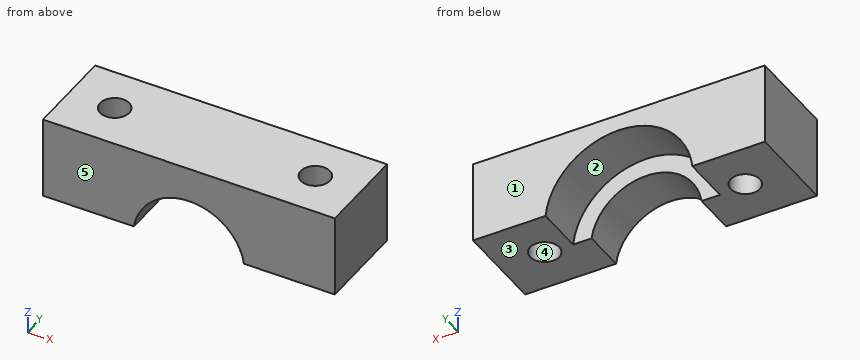
from build123d import *

# Parameters (mm, degrees)
SKETCH1_W           = 32
SKETCH1_H           = 27
SKETCH1_R           = 1.5
BOSS_EXTRUDE1_DEPTH = 25
SKETCH3_W           = 20
SKETCH3_H           = 10
SKETCH3_H_2         = 7
CUT_EXTRUDE1_DEPTH  = 33
SKETCH4_R           = 6.1
CUT_EXTRUDE6_DEPTH  = 18
SKETCH5_R           = 8.1
CUT_EXTRUDE7_DEPTH  = 5.3
SKETCH7_R           = 1.6
CUT_EXTRUDE8_DEPTH  = 26
CUT_EXTRUDE9_DEPTH  = 10
SKETCH10_W          = 32
SKETCH10_H          = 27
CUT_EXTRUDE10_DEPTH = 16


with BuildPart() as part:
    # Sketch1 → Boss-Extrude1 (new body)
    with BuildSketch(Plane.XY):
        with Locations((16, -13.5)):
            Rectangle(SKETCH1_W, SKETCH1_H)
        with Locations((8.5, -3.5)):
            Circle(SKETCH1_R, mode=Mode.SUBTRACT)
        with Locations((23.5, -3.5)):
            Circle(SKETCH1_R, mode=Mode.SUBTRACT)
        with Locations((8.5, -23.5)):
            Circle(SKETCH1_R, mode=Mode.SUBTRACT)
        with Locations((23.5, -23.5)):
            Circle(SKETCH1_R, mode=Mode.SUBTRACT)
    extrude(amount=BOSS_EXTRUDE1_DEPTH)

    # Sketch3 → Cut-Extrude1 (cut, through all)
    with BuildSketch(Plane.ZY):
        with Locations((15, -5)):
            Rectangle(SKETCH3_W, SKETCH3_H)
        with Locations((15, -23.5)):
            Rectangle(SKETCH3_W, SKETCH3_H_2)
    extrude(amount=-CUT_EXTRUDE1_DEPTH, mode=Mode.SUBTRACT)

    # Sketch4 → Cut-Extrude6 (cut, through all)
    with BuildSketch(Plane(origin=(0, -10, 0), x_dir=(1, 0, 0), z_dir=(0, 1, 0))):
        with Locations((15.999687497, -15.1)):
            Circle(SKETCH4_R)
    extrude(amount=-CUT_EXTRUDE6_DEPTH, mode=Mode.SUBTRACT)

    # Sketch5 → Cut-Extrude7 (cut)
    with BuildSketch(Plane(origin=(0, -10, 0), x_dir=(1, 0, 0), z_dir=(0, 1, 0))):
        with Locations((15.999687497, -15.1)):
            Circle(SKETCH5_R)
    extrude(amount=-CUT_EXTRUDE7_DEPTH, mode=Mode.SUBTRACT)

    # Sketch7 → Cut-Extrude8 (cut, through all)
    with BuildSketch(Plane.XY.offset(25)):
        with Locations((5, -15)):
            Circle(SKETCH7_R)
        with Locations((27, -15)):
            Circle(SKETCH7_R)
    extrude(amount=-CUT_EXTRUDE8_DEPTH, mode=Mode.SUBTRACT)

    # Sketch9 → Cut-Extrude9 (cut)
    with BuildSketch(Plane(origin=(0, 0, 0), x_dir=(-1, 0, 0), z_dir=(0, 0, -1))):
        Polygon((-29.138778877, -12.825574808), (-29.952496893, -15.765024245), (-27.813718016, -17.939449437), (-24.861221123, -17.174425192), (-24.047503107, -14.234975755), (-26.186281984, -12.060550563), align=None)
        Polygon((-5, -11.95), (-7.641377482, -13.475), (-7.641377482, -16.525), (-5, -18.05), (-2.358622518, -16.525), (-2.358622518, -13.475), align=None)
    extrude(amount=-CUT_EXTRUDE9_DEPTH, mode=Mode.SUBTRACT)

    # Sketch10 → Cut-Extrude10 (cut)
    with BuildSketch(Plane(origin=(0, 0, 0), x_dir=(-1, 0, 0), z_dir=(0, 0, -1))):
        with Locations((-16, -13.5)):
            Rectangle(SKETCH10_W, SKETCH10_H)
    extrude(amount=-CUT_EXTRUDE10_DEPTH, mode=Mode.SUBTRACT)


solid = part.part
The listing builds one solid part. Answer for the finished solid, in the listing's coordinates (mm). Face numbers are marked on the shaded views. A direction names the side the tool comes from. Round coordinates to 2 decimals unless told otherwise and drop trailing zeros. Write each loop counter-clockwise with the first axis right and the second up, starting at its lowest first coordinate (ties: lowest second). Pieces come first, ordered by that corner, then holes. Notation, with made-up numbers: M 6,40 L 37,40 A20 cw 37,68 Z; hole C -29,0 d8. An arc over 180 degrees is marked long. Write each question's results on one line, items separated by ' | '. Start each with the question number.
Item 1: For a pull along Y with two mould halves and no side action, classify the marked faces 3, 4 and 5 as pulls with the +Y half, pulls with the -Y half, needs draft (parallel to the pull), parting line crosses it, or undercut.
Item 2: For the marked faces 1 and 2, determine the directions among +Z, -Z, +X, -X, +Y, -Y from which every point of the face is accessible in a straight line to the end or side of a thin tool.
Item 3: A flat-ended cylindrical pin translates along its axis: pin 1 Ø3.5 at (x, z) = (17, 19) entering from +Y. Find the tip coordinate at first contact, or state that the pin passes through.
Item 4: A cutting plane is placed at A-A on x = 5. Write down the section's boundary in (y, z), and give its area (3 significant figures).
Item 5: A cutting plane is placed at C-C on y = -13. Write down the section's boundary in (x, z), and give its area (3 significant figures).
Item 6: A cutting plane is placed at B-B on z = 20.5. Write down the section's boundary in (x, y).
Item 7: Straight lines are drawn through the part: L1, parallel to Y at x = 27, z = 21.25; L2, parallel to X at y = -15.75, z = 18; L3, parallel to X at y = -11.5, z = 20.5. For each, find the intervals that lie inside material, in ascending order. Write a range as [from, to].
Item 8: A cutting plane is placed at D-D on z = 22. Write down the section's boundary in (x, y), and give its area (3 significant figures).
Check sheet entries:
1) face 3: needs draft | face 4: undercut | face 5: pulls with the -Y half
2) face 1: +Z, -Z, +X, -X, +Y | face 2: -Z, +Y
3) pin 1: through
4) outline: M -20,16 L -16.6,16 L -16.6,25 L -20,25 Z; M -13.4,16 L -10,16 L -10,25 L -13.4,25 Z | area: 61.2 mm²
5) outline: M 0,16 L 7.95,16 A8.1 cw 24.05,16 L 32,16 L 32,25 L 0,25 Z | area: 199 mm²
6) outline: M 0,-20 L 13.16,-20 L 13.16,-15.3 L 9.96,-15.3 L 9.96,-10 L 0,-10 Z; M 18.84,-20 L 32,-20 L 32,-10 L 22.04,-10 L 22.04,-15.3 L 18.84,-15.3 Z; hole C 5,-15 d3.2; hole C 27,-15 d3.2
7) L1: [-20, -16.6], [-13.4, -10] | L2: [0, 3.59], [6.41, 10.63], [21.37, 25.59], [28.41, 32] | L3: [0, 9.96], [22.04, 32]
8) outline: M 0,-20 L 32,-20 L 32,-10 L 20.24,-10 L 20.24,-15.3 L 11.76,-15.3 L 11.76,-10 L 0,-10 Z; hole C 5,-15 d3.2; hole C 27,-15 d3.2 | area: 259 mm²
